from build123d import *

# Parameters (mm, degrees)
SKETCH_5_W          = 45
SKETCH_5_H          = 22
EXTRUDE_2_DEPTH     = 22
CUT_EXTRUDE_3_DEPTH = 22
CUT_EXTRUDE_START   = 22.5
SKETCH_7_R          = 2.5
CUT_EXTRUDE_4_DEPTH = 10
CUT_EXTRUDE_START_2 = 11
SKETCH_8_R          = 2.5
CUT_EXTRUDE_5_DEPTH = 22
CHAMFER_1_SIZE      = 0.5


with BuildPart() as part:
    # 草图5 → 凸台-拉伸2 (new body)
    with BuildSketch(Plane(origin=(0, 0, 0), x_dir=(1, 0, 0), z_dir=(0, 1, 0))):
        Rectangle(SKETCH_5_W, SKETCH_5_H)
    extrude(amount=EXTRUDE_2_DEPTH)

    # 草图6 → 切除-拉伸3 (cut)
    with BuildSketch(Plane(origin=(0, 0, 0), x_dir=(1, 0, 0), z_dir=(0, 1, 0))):
        with BuildLine():
            Line((-22.5, -1), (-22.5, 1))
            Line((-22.5, 1), (-10.437253933, 1))
            ThreePointArc((-10.437253933, 1), (5.5, 0), (-10.437253933, -1))
            Line((-10.437253933, -1), (-22.5, -1))
        make_face()
    extrude(amount=CUT_EXTRUDE_3_DEPTH, mode=Mode.SUBTRACT)

    # 草图7 → 切除-拉伸4 (cut)
    with BuildSketch(Plane(origin=(0, 0, 0), x_dir=(0, 0, -1), z_dir=(1, 0, 0)).offset(CUT_EXTRUDE_START)):
        with Locations(Location((-6, 17, 0), (0, 0, 180))):
            Circle(SKETCH_7_R)
        with Locations(Location((-6, 5, 0), (0, 0, 180))):
            Circle(SKETCH_7_R)
        with Locations(Location((6, 17, 0), (0, 0, 180))):
            Circle(SKETCH_7_R)
        with Locations(Location((6, 5, 0), (0, 0, 180))):
            Circle(SKETCH_7_R)
    extrude(amount=-CUT_EXTRUDE_4_DEPTH, mode=Mode.SUBTRACT)

    # 草图8 → 切除-拉伸5 (cut)
    with BuildSketch(Plane.XY.offset(CUT_EXTRUDE_START_2)):
        with Locations((-14.5, 11)):
            Circle(SKETCH_8_R)
    extrude(amount=-CUT_EXTRUDE_5_DEPTH, mode=Mode.SUBTRACT)

    # 倒角1
    chamfer_1_edges = [part.edges().sort_by_distance(p)[0] for p in [
        (-22.5, 22, -6),
        (-22.5, 0, 6),
        (-22.5, 22, 6),
        (0, 22, 11),
        (22.5, 22, 0),
        (0, 0, 11),
        (-22.5, 0, -6),
        (0, 0, -11),
        (22.5, 0, 0),
        (22.5, 11, 11),
        (-22.5, 11, 11),
        (-22.5, 11, -11),
        (22.5, 11, -11),
        (0, 22, -11),
    ]]
    chamfer(chamfer_1_edges, length=CHAMFER_1_SIZE)


solid = part.part
Model file for the job. Use its own axes, mm. A direction names the side the tool comes from. Coordinates: 2 decimals unless noted, no trailing zeros. Loops run counter-clockwise (first coordinate to the right, second up) from the corner with the lowest first, then second, coordinate; pieces in that order, holes last. Notation, with made-up numbers: (64, -13.75) -> (112, -13.75) arc R25 ccw to (112, 2.25) -> close; hole circle Ø8 at (75.25, 66). An arc over 180 degrees is marked (long way). Use one line per item in the form item = value. Start each with the question number.
(1) Cut at B-B on x = -18. Give the cut face in (y, z).
(2) Probe probe 1 along Y at (x, z) = (16.5, 6); probe 2 along Z at (x, y) = (19.75, 5); probe 3 along Z at (x, y) = (-11, 13). List the from-to ranges inside material, lowest first. Write a range as from..to.
(3) Cut at A-A on z = -1.5. Give the cut face in (x, y), and give its area (3 significant figures).
(4) Pull direction X, two halves, no side cores. Call faces 1 (the cylindrical face through (5.493, 10.846, -0.338)), 2 (the cylindrical face through (-16, 9, -6)), 3 (the flat face through (12.5, 5, -6)), 4 (the cylindrical face through (17.57, 4.249, -3.615)): pulls with the +X half, pulls with the -X half, needs draft (parallel to the pull), parting line crosses it, or undercut.
(5) Cut at C-C on x = 13.5. Give the cut face in (y, z), and give its area (3 significant figures).
(6) Flat gauge pins, fed straight in: pin 1 (6 mm diameter, centred on x = -14.5, y = 11, fed in from +Z); pin 2 (2.5 mm diameter, centred on y = 17.5, z = 5.5, fed in from +X); pin 3 (13 mm diameter, centred on x = -2.5, z = 0, fed in from -Y). Where does each tip first touch, or does it go through?
(7) Tool access for faces 5 (the flat face through (-18, 11, 1)), 6 (the cylindrical face through (17.57, 4.249, 8.385)), 7 (the flat face through (22.5, 11, 0)): list every direction of +Z, -Z, +X, -X, +Y, -Y with a clear straight run to the whole face (end or side of a thin tool).
(8) Cut at D-D on z = 4.25. Give the cut face in (x, y).
Values:
q1.outline = (0, -10.5) -> (0.5, -11) -> (21.5, -11) -> (22, -10.5) -> (22, -1) -> (0, -1) -> close; (0, 1) -> (22, 1) -> (22, 10.5) -> (21.5, 11) -> (0.5, 11) -> (0, 10.5) -> close
q2.probe_1 = 0..2.5, 7.5..14.5, 19.5..22
q2.probe_2 = -11..-8.5, -3.5..3.5, 8.5..11
q2.probe_3 = -11..-1, 1..11
q3.outline = (-22.5, 0.5) -> (-22, 0) -> (-10.36, 0) -> (-10.36, 22) -> (-22, 22) -> (-22.5, 21.5) -> close; (5.36, 0) -> (22, 0) -> (22.5, 0.5) -> (22.5, 21.5) -> (22, 22) -> (5.36, 22) -> close; hole circle Ø5 at (-14.5, 11)
q3.area = 624 mm2
q4.face_1 = undercut
q4.face_2 = undercut
q4.face_3 = pulls with the +X half
q4.face_4 = needs draft
q5.outline = (0, -10.5) -> (0.5, -11) -> (21.5, -11) -> (22, -10.5) -> (22, 10.5) -> (21.5, 11) -> (0.5, 11) -> (0, 10.5) -> close; hole circle Ø5 at (5, -6); hole circle Ø5 at (5, 6); hole circle Ø5 at (17, -6); hole circle Ø5 at (17, 6)
q5.area = 405 mm2
q6.pin_1 = 11
q6.pin_2 = 12.5
q6.pin_3 = through
q7.face_5 = -X, +Y, -Y
q7.face_6 = +X
q7.face_7 = +Z, -Z, +X, +Y, -Y
q8.outline = (-22.5, 0.5) -> (-22, 0) -> (-9.28, 0) -> (-9.28, 22) -> (-22, 22) -> (-22.5, 21.5) -> close; (4.28, 0) -> (22, 0) -> (22.5, 0.5) -> (22.5, 3.21) -> (12.5, 3.21) -> (12.5, 6.79) -> (22.5, 6.79) -> (22.5, 15.21) -> (12.5, 15.21) -> (12.5, 18.79) -> (22.5, 18.79) -> (22.5, 21.5) -> (22, 22) -> (4.28, 22) -> close; hole circle Ø5 at (-14.5, 11)
